The listing builds one solid part. Answer for the finished solid, in the listing's coordinates (mm). A direction names the side the tool comes from. Give positions to 0.01 mm unless a question says otherwise; leave off trailing zeros. Order: outer loops, then holes, each group sorted by start corner. A loop starts at its lowest first (then second) coordinate and runs counter-clockwise, first axis right, second up. Notation, with made-up numbers: (51.5, 23.5) - (90.5, 23.5) arc R20 ccw to (90.5, 47.5) - close; hole circle Ø10 at (-25.75, 12). An arc over 180 degrees is marked (long way). Answer as a JSON object with one key per item and string values. Group by question number.
Q1. A cutting plane is placed at B-B, the plane x = -2.25. Give the vertices of the cut face in (y, z), and give its area (3 significant figures).
Q2. For faces 5 (the face through (2, 18, 78)), 6 (the face through (-2, 29, 10)), 7 (the face through (3, 18, 73)), 8 (the face through (-2, 29, 55)), 9 (the face through (-3, 19, 60)), determine the directions among +Z, -Z, +X, -X, +Y, -Y from which every point of the face is accessible in a straight line to the end or side of a thin tool.
Q3. A cutting plane is placed at D-D, the plane z = 33. Give the vertices of the cut face in (x, y).
Q4. The mould has two halves that part along Z. Classify faces 1 (the face through (-1, 23.915, 60)), 2 (the face through (1, 18, 80)), 3 (the face through (2, 18, 39)), 4 (the face through (-2, 28, 20)): released by +Z, released by -Z, zero draft, split by the parting line, or undercut.
Q5. A cutting plane is placed at A-A, the plane y = 23. Give the vertices of the cut face in (x, z), and give its area (3 significant figures).
Q6. Consider line 1 (Z direction, x = 3, y = 14); line 2 (X direction, y = 15, z = 11.5); line 3 (Z direction, x = -3, y = 27.5). Determine where each line is inside the solid, lowest interval first.
Q7. Given pin 1 (0.8 mm diameter, centred on x = -3.5, z = 13.5, fed in from -Y); pin 2 (2 mm diameter, centred on x = 3.5, y = 23, fed in from +Z); pin 3 (3 mm diameter, centred on x = -2, y = 24.5, fed in from -Z), each flat-ended and moving along its own axis, determine where each tip first touches the part or whether it passes through.
Solid Edge part; units mm, degrees
sketch "Sketch1" plane through (0, 0, 0) normal (-1, 0, 0) x (0, -1, 0)
  line L0 (2.0853, 0) -> (2.0853, 80)
  line L1 (2.0853, 80) -> (-37.9147, 80)
  line L2 (-37.9147, 80) -> (-37.9147, 0)
  line L3 (-37.9147, 0) -> (2.0853, 0)
extrude "Protrusion1" add sketch "Sketch1" against normal blind 2
sketch "Sketch2" plane through (0, 18.9573, 40) normal (-1, 0, 0) x (0, 0, 1)
  line L0 (-20, 4.9573) -> (-20, 18.9573)
  line L1 (-30, 18.9573) -> (-20, 18.9573)
  line L2 (-30, 18.9573) -> (-30, 4.9573)
  line L3 (-30, 4.9573) -> (-20, 4.9573)
  line L4 (25, 18.9573) -> (25, 4.9573)
  line L5 (25, 4.9573) -> (15, 4.9573)
  line L6 (15, 4.9573) -> (15, 18.9573)
  line L7 (15, 18.9573) -> (25, 18.9573)
extrude "Vysunutí_2" add sketch "Sketch2" along normal blind 3
sketch "Sketch3" plane through (-3, 30.9147, 60) normal (-1, 0, 0) x (0, 0, 1)
  line L0 (5, -17) -> (5, 7)
  line L1 (5, 7) -> (-5, 7)
  line L2 (-5, 7) -> (-5, -17)
  line L3 (-5, -17) -> (5, -17)
  line L4 (-40, -17) -> (-40, 7)
  line L5 (-40, 7) -> (-50, 7)
  line L6 (-50, 7) -> (-50, -17)
  line L7 (-50, -17) -> (-40, -17)
extrude "Vysunutí_3" add sketch "Sketch3" along normal blind 1
sketch "Sketch4" plane through (2, 17.9147, 40) normal (1, 0, 0) x (0, 0, 1)
  line L0 (33, 20) -> (33, -20)
  line L1 (33, -20) -> (35, -20)
  line L2 (35, -20) -> (35, 20)
  line L3 (35, 20) -> (33, 20)
extrude "Protrusion2" add sketch "Sketch4" along normal blind 2
sketch "Sketch5" plane through (2, 17.9147, 36.5) normal (1, 0, 0) x (0, 0, -1)
  line L0 (31.5, 20) -> (31.5, -20)
  line L1 (31.5, -20) -> (33.5, -20)
  line L2 (33.5, -20) -> (33.5, 20)
  line L3 (33.5, 20) -> (31.5, 20)
extrude "Vysunutí_6" add sketch "Sketch5" along normal blind 2
sketch "Sketch6" plane through (2, 17.9147, 39) normal (1, 0, 0) x (0, -1, 0)
  line L0 (19, 39) -> (19, -41)
  line L1 (19, -41) -> (20, -41)
  line L2 (20, -41) -> (20, 39)
  line L3 (20, 39) -> (19, 39)
extrude "Vyříznutí_1" cut sketch "Sketch6" against normal blind 2
sketch "Sketch7" plane through (2, 17.9147, 39) normal (1, 0, 0) x (0, -1, 0)
  line L0 (20, -41) -> (20, 39)
  line L1 (20, 39) -> (19, 39)
  line L2 (19, 39) -> (19, -41)
  line L3 (19, -41) -> (20, -41)
extrude "Vyříznutí_2" cut sketch "Sketch7" along normal blind 2
Reply:
{
 "1": {"outline": "(23.91, 10) - (37.91, 10) - (37.91, 20) - (23.91, 20) - close; (23.91, 55) - (37.91, 55) - (37.91, 65) - (23.91, 65) - close", "area": "280 mm^2"},
 "2": {"face 5": "+Z, +X, +Y, -Y", "face 6": "-Z, -X, +Y, -Y", "face 7": "+X, +Y, -Y", "face 8": "-X, +Y, -Y", "face 9": "+Z, -Z, -Y"},
 "3": {"outline": "(0, -1.09) - (2, -1.09) - (2, 37.91) - (0, 37.91) - close"},
 "4": {"face 1": "zero draft", "face 2": "released by +Z", "face 3": "undercut", "face 4": "undercut"},
 "5": {"outline": "(-4, 10) - (-3, 10) - (-3, 20) - (-4, 20) - close; (-4, 55) - (-3, 55) - (-3, 65) - (-4, 65) - close; (0, 0) - (2, 0) - (2, 3) - (4, 3) - (4, 5) - (2, 5) - (2, 73) - (4, 73) - (4, 75) - (2, 75) - (2, 80) - (0, 80) - close", "area": "188 mm^2"},
 "6": {"line 1": "z = 3 to 5, 73 to 75", "line 2": "x = -4 to -3, 0 to 2", "line 3": "z = 10 to 20, 55 to 65"},
 "7": {"pin 1": "stops at y = 13.91", "pin 2": "stops at z = 75", "pin 3": "stops at z = 10"}
}
